Build history of the part. All positions in model axes, mm. A direction names the side the tool comes from. Round coordinates to 2 decimals unless told otherwise and drop trailing zeros. Order: outer loops, then holes, each group sorted by start corner. A loop starts at its lowest first (then second) coordinate and runs counter-clockwise, first axis right, second up. Notation, with made-up numbers: (-5.5, 76) -> (3.5, 76) arc R25 cw to (3.5, 105) -> close; hole circle Ø8 at (25.5, -35). An arc over 180 degrees is marked (long way). Answer as a JSON object with one key per item and string values.
from build123d import *

# Parameters (mm, degrees)
SKETCH1_W           = 202
SKETCH1_H           = 72
BOSS_EXTRUDE1_DEPTH = 29
SKETCH2_W           = 199
SKETCH2_H           = 69
CUT_EXTRUDE1_DEPTH  = 27
SKETCH3_W           = 185
SKETCH3_H           = 37
CUT_EXTRUDE2_DEPTH  = 27
FILLET1_R           = 6
FILLET2_R           = 4.5
FILLET3_R           = 6
SKETCH4_W           = 4
SKETCH4_H           = 29
BOSS_EXTRUDE2_DEPTH = 1
FILLET4_R           = 2
FILLET5_R           = 3


with BuildPart() as part:
    # Sketch1 → Boss-Extrude1 (new body)
    with BuildSketch(Plane.XY):
        with Locations((101, 36)):
            Rectangle(SKETCH1_W, SKETCH1_H)
    extrude(amount=BOSS_EXTRUDE1_DEPTH)

    # Sketch2 → Cut-Extrude1 (cut)
    with BuildSketch(Plane.XY.offset(29)):
        with Locations((101, 36)):
            Rectangle(SKETCH2_W, SKETCH2_H)
    extrude(amount=-CUT_EXTRUDE1_DEPTH, mode=Mode.SUBTRACT)

    # Sketch3 → Cut-Extrude2 (cut)
    with BuildSketch(Plane.XY.offset(2)):
        with Locations((101, 36.5)):
            Rectangle(SKETCH3_W, SKETCH3_H)
    extrude(amount=-CUT_EXTRUDE2_DEPTH, mode=Mode.SUBTRACT)

    # Fillet1
    fillet1_edges = [part.edges().sort_by_distance(p)[0] for p in [
        (8.5, 18, 1),
        (8.5, 55, 1),
        (193.5, 55, 1),
        (193.5, 18, 1),
    ]]
    fillet(fillet1_edges, radius=FILLET1_R)

    # Fillet2
    fillet2_edges = [part.edges().sort_by_distance(p)[0] for p in [
        (1.5, 1.5, 15.5),
        (1.5, 70.5, 15.5),
        (200.5, 70.5, 15.5),
        (200.5, 1.5, 15.5),
    ]]
    fillet(fillet2_edges, radius=FILLET2_R)

    # Fillet3
    fillet3_edges = [part.edges().sort_by_distance(p)[0] for p in [
        (0, 72, 14.5),
        (202, 72, 14.5),
        (202, 0, 14.5),
        (0, 0, 14.5),
    ]]
    fillet(fillet3_edges, radius=FILLET3_R)

    # Sketch4 → Boss-Extrude2 (add)
    with BuildSketch(Plane(origin=(0, 0, 0), x_dir=(-1, 0, 0), z_dir=(0, -1, 0))):
        with Locations((-23, -14.5)):
            Rectangle(SKETCH4_W, SKETCH4_H)
        with Locations((-179, -14.5)):
            Rectangle(SKETCH4_W, SKETCH4_H)
    extrude(amount=BOSS_EXTRUDE2_DEPTH)

    # Fillet4
    fillet4_edges = [part.edges().sort_by_distance(p)[0] for p in [
        (200.242640687, 1.757359313, 0),
        (188.5, 0, 0),
        (202, 36, 0),
        (0, 36, 0),
        (101, 72, 0),
        (13.5, 0, 0),
        (1.757359313, 70.242640687, 0),
        (1.757359313, 1.757359313, 0),
        (200.242640687, 70.242640687, 0),
    ]]
    fillet(fillet4_edges, radius=FILLET4_R)

    # Fillet5
    fillet5_edges = [part.edges().sort_by_distance(p)[0] for p in [
        (101, 70.5, 2),
        (200.5, 36, 2),
        (1.5, 36, 2),
        (101, 1.5, 2),
        (2.818019485, 69.181980515, 2),
        (2.818019485, 2.818019485, 2),
        (199.181980515, 2.818019485, 2),
        (199.181980515, 69.181980515, 2),
    ]]
    fillet(fillet5_edges, radius=FILLET5_R)


solid = part.part
1) Cut at B-B, the plane z = 24.75. Give the cut face in (x, y).
Checked values:
{"outline": "(0, 6) arc R6 ccw to (6, 0) -> (21, 0) -> (21, -1) -> (25, -1) -> (25, 0) -> (177, 0) -> (177, -1) -> (181, -1) -> (181, 0) -> (196, 0) arc R6 ccw to (202, 6) -> (202, 66) arc R6 ccw to (196, 72) -> (6, 72) arc R6 ccw to (0, 66) -> close; hole (1.5, 6) arc R4.5 ccw to (6, 1.5) -> (196, 1.5) arc R4.5 ccw to (200.5, 6) -> (200.5, 66) arc R4.5 ccw to (196, 70.5) -> (6, 70.5) arc R4.5 ccw to (1.5, 66) -> close"}
2) Cut at A-A, the plane x = 175. Give the cut face in (y, z).
Checked values:
{"outline": "(0, 0) -> (18, 0) -> (18, 2) -> (4.5, 2) arc R3 cw to (1.5, 5) -> (1.5, 29) -> (0, 29) -> close; (55, 0) -> (70, 0) arc R2 ccw to (72, 2) -> (72, 29) -> (70.5, 29) -> (70.5, 5) arc R3 cw to (67.5, 2) -> (55, 2) -> close"}
3) Pull direction X, two halves, no side cores. Call faces 4 (the face through (100, 70.5, 17)), 5 (the face through (100, 0, 14)), 6 (the face through (23, -1, 14)), 7 (the face through (1.711, 1.804, 15.689)): pulls with the +X half, pulls with the -X half, needs draft (parallel to the pull), parting line crosses it, or undercut.
Checked values:
{"face 4": "undercut", "face 5": "undercut", "face 6": "needs draft", "face 7": "pulls with the -X half"}
4) Which spindle directions (+Z, -Z, +X, -X, +Y, -Y) get a long thin tool onto all of the face, cutting with end or side? Do faces 1 (the face through (188, 0, 15)), 2 (the face through (191.789, 53.196, 0.986)), 3 (the face through (199.147, 69.217, 16.832)). Say none if no direction does.
Checked values:
{"face 1": "+Z, -Z, +X, -Y", "face 2": "+Z, -Z", "face 3": "+Z"}
5) Probe L1, parallel to Y at x = 68.5, z = 8; L2, parallel to X at y = 50, z = 16.75; L3, parallel to Z at x = 100, y = 61. List the from-to ranges inside material, lowest first. Write a range as from..to.
Checked values:
{"L1": "y = 0..1.5, 70.5..72", "L2": "x = 0..1.5, 200.5..202", "L3": "z = 0..2"}
6) Cut at D-D, the plane y = 8. Give the cut face in (x, z).
Checked values:
{"outline": "(0, 2) arc R2 ccw to (2, 0) -> (200, 0) arc R2 ccw to (202, 2) -> (202, 29) -> (200.5, 29) -> (200.5, 5) arc R3 cw to (197.5, 2) -> (4.5, 2) arc R3 cw to (1.5, 5) -> (1.5, 29) -> (0, 29) -> close"}
7) Cut at C-C, the plane y = 21. Give the cut face in (x, z), plus the area to 3 significant figures.
Checked values:
{"outline": "(0, 2) arc R2 ccw to (2, 0) -> (9.3, 0) -> (9.3, 2) -> (4.5, 2) arc R3 cw to (1.5, 5) -> (1.5, 29) -> (0, 29) -> close; (192.7, 0) -> (200, 0) arc R2 ccw to (202, 2) -> (202, 29) -> (200.5, 29) -> (200.5, 5) arc R3 cw to (197.5, 2) -> (192.7, 2) -> close", "area": "120 mm²"}
8) Flat gauge pins, fed straight in: pin 1 Ø12 at (x, z) = (192, 20.5) entering from -Y; pin 2 Ø1.5 at (y, z) = (1, 8) entering from -X; pin 3 Ø0.6 at (x, z) = (88.5, 1) entering from +Y. Where does each tip first touch, or does it go through?
Checked values:
{"pin 1": "stops at y = 0", "pin 2": "stops at x = 1.76", "pin 3": "stops at y = 71.87"}
